```python
from build123d import *

# Parameters (mm, degrees)
BASPROSKE_W        = 6.35
BASPROSKE_H        = 17
TOOTHCUT_DEPTH     = 25.86609137
TEETHCUTS_COUNT    = 15
BORSKE_R           = 0.4
BORE_DEPTH         = 50.0000508
CUT_EXTRUDE1_DEPTH = 25.830915598


with BuildPart() as part:
    # BasProSke → Base-Revolve (revolve)
    with BuildSketch(Plane(origin=(0, 0, 0), x_dir=(1, 0, 0), z_dir=(0, 1, 0)), mode=Mode.PRIVATE) as base_revolve_sk:
        with Locations((3.175, 8.5)):
            Rectangle(BASPROSKE_W, BASPROSKE_H)
    revolve(base_revolve_sk.sketch.rotate(Axis((-10, 0, 0), (1, 0, 0)), 180), axis=Axis((-10, 0, 0), (1, 0, 0)))

    # TooCutSke → ToothCut (cut, through all)
    with BuildSketch(Plane(origin=(0, 0, 0), x_dir=(0, 0, -1), z_dir=(1, 0, 0))):
        with BuildLine():
            ThreePointArc((1.050056448, 12.454813626), (0, 12.499), (-1.050056448, 12.454813626))
            ThreePointArc((-1.050056448, 12.454813626), (-1.638118106, 14.809604533), (-3.110934279, 16.73876737))
            ThreePointArc((-3.110934279, 16.73876737), (0, 17.0254), (3.110934279, 16.73876737))
            ThreePointArc((3.110934279, 16.73876737), (1.638118106, 14.809604533), (1.050056448, 12.454813626))
        make_face()
    toothcut = extrude(amount=TOOTHCUT_DEPTH, mode=Mode.SUBTRACT)

    # TeethCuts: ToothCut ×15 about axis
    teethcuts_axis = Axis((0, 0, 0), (1, 0, 0))
    for i in range(1, TEETHCUTS_COUNT):
        add(toothcut.rotate(teethcuts_axis, i * 360 / TEETHCUTS_COUNT), mode=Mode.SUBTRACT)

    # BorSke → Bore (cut, symmetric)
    with BuildSketch(Plane(origin=(0, 0, 0), x_dir=(0, 0, -1), z_dir=(1, 0, 0))):
        with Locations(Location((0, 0, 0), (0, 0, 180))):
            Circle(BORSKE_R)
    extrude(amount=BORE_DEPTH, both=True, mode=Mode.SUBTRACT)

    # Sketch1 → Cut-Extrude1 (cut, through all)
    with BuildSketch(Plane.ZY):
        with BuildLine():
            Line((1.659895813, 1.69164), (-1.659895813, 1.69164))
            ThreePointArc((-1.659895813, 1.69164), (-0.917318626, -2.185274934), (2.37, 0))
            ThreePointArc((2.37, 0), (2.185274934, 0.917318626), (1.659895813, 1.69164))
        make_face()
    extrude(amount=-CUT_EXTRUDE1_DEPTH, mode=Mode.SUBTRACT)


solid = part.part
```
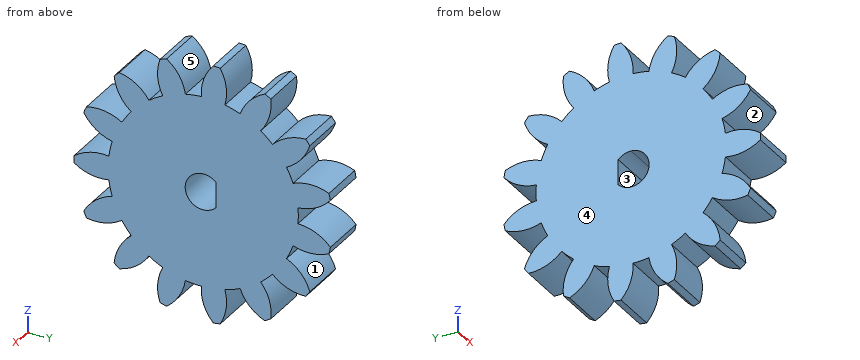
Check sheet for the modelled part. Datum: model origin and axes. Units: mm. Face numbers are marked on the shaded views. A direction names the side the tool comes from. Give positions to 0.01 mm unless a question says otherwise; leave off trailing zeros. Loops run counter-clockwise (first coordinate to the right, second up) from the corner with the lowest first, then second, coordinate; pieces in that order, holes last. Notation, with made-up numbers: M 56.5,-24 L 90.5,-24 A21 cw 90.5,14 Z; hole C 29,68.25 d10. An arc over 180 degrees is marked long. Answer in a Markdown table with one row per item.
1) Tool access check on the marked faces 1, 2, 3, 4 and 5. Record the directions out of +Z, -Z, +X, -X, +Y, -Y that give a thin tool (end or side, any length) a straight path to the whole face; none if there is none.
Solutions:
| item | result |
|---|---|
| face 1 | +X, -X, +Y |
| face 2 | +X, -X, -Y |
| face 3 | +X, -X |
| face 4 | +Z, -Z, -X, +Y, -Y |
| face 5 | +Z, +X, -X |
2) Thickness scan on line 1 (Y direction, x = 1.5, z = 0); line 2 (Y direction, x = 3.5, z = 13); line 3 (Z direction, x = 0.5, y = 13). Record the ranges inside material, lowest first.
Solutions:
| item | result |
|---|---|
| line 1 | y = -17 to -2.37, 1.69 to 12.5 |
| line 2 | y = -5.9 to -2.5, -0.27 to 3.02, 5.65 to 8.88 |
| line 3 | z = -10.35 to -7.69, -4.44 to -1.1, 1.1 to 4.44, 7.69 to 10.35 |
3) Cross-section at B-B (y = 15). Enter the section's corners in (x, z).
Solutions:
| item | result |
|---|---|
| outline | M 0,-4.45 L 6.35,-4.45 L 6.35,-1.73 L 0,-1.73 Z; M 0,1.73 L 6.35,1.73 L 6.35,4.45 L 0,4.45 Z |
4) Depth check by flat-ended pin: pin 1 (3 mm diameter, centred on x = 1, z = -13, fed in from -Y); pin 2 (3 mm diameter, centred on x = 3, y = -10.5, fed in from +Z). Enter the tip coordinate at first touch or a pass-through.
Solutions:
| item | result |
|---|---|
| pin 1 | stops at y = -11.71 |
| pin 2 | stops at z = 12.93 |
5) Cross-section at C-C (y = -14.5). Enter the section's corners in (x, z), plus the area to 3 significant figures.
Solutions:
| item | result |
|---|---|
| outline | M 0,-7.46 L 6.35,-7.46 L 6.35,-4.98 L 0,-4.98 Z; M 0,-1.55 L 6.35,-1.55 L 6.35,1.55 L 0,1.55 Z; M 0,4.98 L 6.35,4.98 L 6.35,7.46 L 0,7.46 Z |
| area | 51.1 mm^2 |
6) Cross-section at D-D (y = -3). Enter the section's corners in (x, z).
Solutions:
| item | result |
|---|---|
| outline | M 0,-14.25 L 6.35,-14.25 L 6.35,14.25 L 0,14.25 Z |
7) Cross-section at A-A (z = 0). Enter the section's corners in (x, y), plus the area to 3 significant figures.
Solutions:
| item | result |
|---|---|
| outline | M 0,-17 L 6.35,-17 L 6.35,-2.37 L 0,-2.37 Z; M 0,1.69 L 6.35,1.69 L 6.35,12.5 L 0,12.5 Z |
| area | 162 mm^2 |
